Check sheet for the modelled part. Datum: model origin and axes. Units: mm. Give positions to 0.01 mm unless a question says otherwise; leave off trailing zeros. Loops run counter-clockwise (first coordinate to the right, second up) from the corner with the lowest first, then second, coordinate; pieces in that order, holes last. Notation, with made-up numbers: (-16, -26) -> (40, -26) arc R24 cw to (40, 3) -> close; hole circle Ø8 at (72.5, 67.5). An arc over 180 degrees is marked (long way). Write each question's results on one line, items separated by ' | '. Start each with the question number.
1. Material ranges on L1, parallel to X at y = 241.3, z = 0.25; L2, parallel to Y at x = 12.7, z = 0.25; L3, parallel to Y at x = 100, z = -1.75, recorded low to high. Write a range as from..to.
2. Cross-section at B-B on y = 12.7. Record the boundary of the cut face in (x, z) (3 decimals).
3. Gauge pin test, flat ends, axial feed: pin 1 Ø4.5 at (x, y) = (101.6, 12.7) entering from +Z; pin 2 Ø8 at (x, y) = (12.7, 241.3) entering from -Z (3 decimals). Record the tip position at first contact, or that the pin passes through.
4. Cross-section at A-A on x = 12.7. Record the boundary of the cut face in (y, z) (3 decimals), and give its area (3 significant figures).
5. Mould release check, pull along Y, two halves, no side actions. Record for faces 1 (the face through (12.38, 15.17, 0.04)), 2 (the face through (56, 0, 0)), 3 (the face through (0, 125, 0)), 4 (the face through (56, 254, 0)): +Y half, -Y half, draft (parallel to the pull), parting line (faces both ways), or undercut.
from build123d import *

# Parameters (mm, degrees)
SKETCH1_W           = 114.3
SKETCH1_H           = 254
BOSS_EXTRUDE1_DEPTH = 3.175
SKETCH2_R           = 2.4892
CUT_EXTRUDE1_DEPTH  = 279.6051193


with BuildPart() as part:
    # Sketch1 → Boss-Extrude1 (new, symmetric)
    with BuildSketch(Plane.XY):
        with Locations((57.15, 127)):
            Rectangle(SKETCH1_W, SKETCH1_H)
    extrude(amount=BOSS_EXTRUDE1_DEPTH, both=True)

    # Sketch2 → Cut-Extrude1 (cut, through all)
    with BuildSketch(Plane.XY.offset(3.175)):
        with Locations((12.7, 241.3)):
            Circle(SKETCH2_R)
        with Locations((12.7, 12.7)):
            Circle(SKETCH2_R)
        with Locations((101.6, 241.3)):
            Circle(SKETCH2_R)
        with Locations((101.6, 12.7)):
            Circle(SKETCH2_R)
    extrude(amount=-CUT_EXTRUDE1_DEPTH, mode=Mode.SUBTRACT)


solid = part.part
Geometry says:
1) L1: 0..10.21, 15.19..99.11, 104.09..114.3 | L2: 0..10.21, 15.19..238.81, 243.79..254 | L3: 0..10.79, 14.61..239.39, 243.21..254
2) outline: (0, -3.175) -> (10.211, -3.175) -> (10.211, 3.175) -> (0, 3.175) -> close; (15.189, -3.175) -> (99.111, -3.175) -> (99.111, 3.175) -> (15.189, 3.175) -> close; (104.089, -3.175) -> (114.3, -3.175) -> (114.3, 3.175) -> (104.089, 3.175) -> close
3) pin 1: through | pin 2: z = -3.175
4) outline: (0, -3.175) -> (10.211, -3.175) -> (10.211, 3.175) -> (0, 3.175) -> close; (15.189, -3.175) -> (238.811, -3.175) -> (238.811, 3.175) -> (15.189, 3.175) -> close; (243.789, -3.175) -> (254, -3.175) -> (254, 3.175) -> (243.789, 3.175) -> close | area: 1,550 mm^2
5) face 1: undercut | face 2: -Y half | face 3: draft | face 4: +Y half
